Could you check a few things on this drawing? It's one solid part, dimensions in mm from its lowest x, y, z. A direction names the side the tool comes from. Give positions to 0.01 mm unless a question says otherwise; leave off trailing zeros. Loops run counter-clockwise (first coordinate to the right, second up) from the corner with the lowest first, then second, coordinate; pieces in that order, holes last.
Q1. I need wall thicknesses on probe 1 along X at (y, z) = (6, 1.75); probe 2 along X at (y, z) = (4, 2.95); probe 3 along Y at (x, z) = (11.5, 0.6). Which ranges of each line are inside material? Lowest first, please.
Q2. Suppose I cut it at A-A (x = 5.25). List the corners of the cut face in (y, z) for me (3 decimals), and give its area (3 significant figures).
Q3. For the marked faces 1 and 2, which set-ups out of +Z, -Z, +X, -X, +Y, -Y let a thin tool reach every point of the face, with its end or its side?
Q4. Suppose I cut it at B-B (z = 1.75). List the corners of the cut face in (x, y) for me.
Q5. Thinking about a two-plate mould opening in X: for the marked faces 3, 4 and 5, which applies, pulls with the +X half, pulls with the -X half, needs draft (parallel to the pull), parting line crosses it, or undercut?
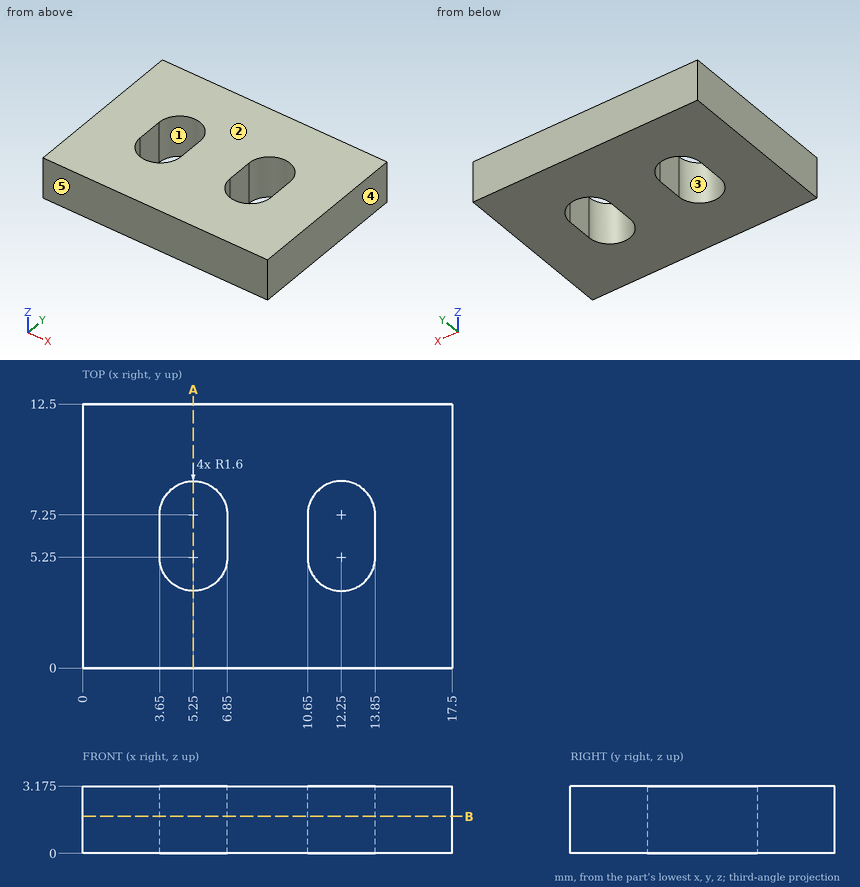
Solutions:
1. probe 1: x = 0 to 3.65, 6.85 to 10.65, 13.85 to 17.5
1. probe 2: x = 0 to 4.25, 6.25 to 11.25, 13.25 to 17.5
1. probe 3: y = 0 to 3.84, 8.66 to 12.5
2. outline: (0, 0) - (3.65, 0) - (3.65, 3.175) - (0, 3.175) - close; (8.85, 0) - (12.5, 0) - (12.5, 3.175) - (8.85, 3.175) - close
2. area: 23.2 mm2
3. face 1: +Z, -Z
3. face 2: +Z, +X, -X, +Y, -Y
4. outline: (0, 0) - (17.5, 0) - (17.5, 12.5) - (0, 12.5) - close; hole (3.65, 5.25) arc R1.6 ccw to (6.85, 5.25) - (6.85, 7.25) arc R1.6 ccw to (3.65, 7.25) - close; hole (10.65, 5.25) arc R1.6 ccw to (13.85, 5.25) - (13.85, 7.25) arc R1.6 ccw to (10.65, 7.25) - close
5. face 3: undercut
5. face 4: pulls with the +X half
5. face 5: needs draft
